```python
from build123d import *

# Parameters (mm, degrees)
SKETCH_4_W                   = 147
SKETCH_4_H                   = 102
EXTRUDE_1_DEPTH              = 26.5
PATTERN_LINEAR_3_COUNT       = 2
PATTERN_LINEAR_3_PITCH       = 44.45
PATTERN_LINEAR_3_COUNT_DIR2  = 2
PATTERN_LINEAR_3_PITCH_DIR2  = 95
SKETCH_10_W                  = 9
SKETCH_10_H                  = 5
CUT_EXTRUDE_1_DEPTH          = 103
SKETCH_12_W                  = 19.5
SKETCH_12_H                  = 5
CUT_EXTRUDE_2_DEPTH          = 103
CUT_EXTRUDE_3_DEPTH          = 4
CUT_EXTRUDE_4_DEPTH          = 1
CUT_EXTRUDE_7_DEPTH          = 5
SKETCH_16_W                  = 6
SKETCH_16_H                  = 3
CUT_EXTRUDE_8_DEPTH          = 4
PATTERN_LINEAR_4_COUNT       = 2
PATTERN_LINEAR_4_PITCH       = 41.61
PATTERN_LINEAR_4_COL_COUNT   = 2
PATTERN_LINEAR_4_COL_PITCH   = 101.6
MIRROR_2_COPY_1_SKETCH_W     = 6
MIRROR_2_COPY_1_SKETCH_H     = 3
MIRROR_2_COPY_1_DEPTH        = 4
MIRROR_2_COPY_2_SKETCH_W     = 6
MIRROR_2_COPY_2_SKETCH_H     = 3
MIRROR_2_COPY_2_DEPTH        = 4
PATTERN_LINEAR_1_COUNT       = 2
PATTERN_LINEAR_1_PITCH       = 41.61
PATTERN_LINEAR_1_COL_COUNT   = 2
PATTERN_LINEAR_1_COL_PITCH   = 101.6
SKETCH_17_R                  = 2.5
EXTRUDE_2_DEPTH              = 3
PATTERN_LINEAR_5_COUNT       = 2
PATTERN_LINEAR_5_PITCH       = 46.5
SKETCH_18_R                  = 2.5
EXTRUDE_3_DEPTH              = 3
DRAFT_1_ANGLE                = 2
SKETCH_19_W                  = 9
SKETCH_19_H                  = 81
CUT_EXTRUDE_9_DEPTH          = 1
SKETCH_21_W                  = 9
SKETCH_21_H                  = 42
CUT_EXTRUDE_10_DEPTH         = 4
SKETCH_22_W                  = 7
SKETCH_22_H                  = 41
SKETCH_22_H_2                = 40.5
CUT_EXTRUDE_11_DEPTH         = 6
HOLE_WIZARD_M3_3_D           = 2.5
HOLE_WIZARD_M3_3_DEPTH       = 8.5
HOLE_WIZARD_M3_3_CSINK_D     = 3.05
HOLE_WIZARD_M3_3_CSINK_ANGLE = 90
HOLE_WIZARD_M3_3_TIP         = 0.751075774
FILLET_1_R                   = 4


with BuildPart() as part:
    # 草图4 → 凸台-拉伸1 (new body)
    with BuildSketch(Plane(origin=(0, 0, 0), x_dir=(1, 0, 0), z_dir=(0, 1, 0))):
        Rectangle(SKETCH_4_W, SKETCH_4_H)
    extrude(amount=EXTRUDE_1_DEPTH)

    # 草图9 → M3 螺纹孔2 (revolve, cut)
    with BuildSketch(Plane(origin=(32.22, 0, 47.5), x_dir=(0, 0, -1), z_dir=(1, 0, 0))):
        Polygon((0, 0), (0, 8.251075774), (1.25, 7.5), (1.25, 0.275), (1.525, 0), align=None)
    hole_wizard_m3_2 = revolve(axis=Axis((32.22, -6.35, 47.5), (0, 1, 0)), mode=Mode.SUBTRACT)

    # 阵列(线性)3: Hole Wizard M3 _2 2 × 2
    with Locations(*[(-i * PATTERN_LINEAR_3_PITCH, 0, -j * PATTERN_LINEAR_3_PITCH_DIR2) for i in range(PATTERN_LINEAR_3_COUNT) for j in range(PATTERN_LINEAR_3_COUNT_DIR2) if (i, j) != (0, 0)]):
        add(hole_wizard_m3_2, mode=Mode.SUBTRACT)

    # 草图10 → 切除-拉伸1 (cut, through all)
    with BuildSketch(Plane.XY.offset(51)):
        with Locations((-69, 2.5)):
            Rectangle(SKETCH_10_W, SKETCH_10_H)
    extrude(amount=-CUT_EXTRUDE_1_DEPTH, mode=Mode.SUBTRACT)

    # 草图12 → 切除-拉伸2 (cut, through all)
    with BuildSketch(Plane.XY.offset(51)):
        with Locations((63.75, 2.5)):
            Rectangle(SKETCH_12_W, SKETCH_12_H)
    extrude(amount=-CUT_EXTRUDE_2_DEPTH, mode=Mode.SUBTRACT)

    # 草图13 → 切除-拉伸3 (cut)
    with BuildSketch(Plane.XZ.offset(-5)):
        Polygon((54, -51), (73.5, -31.5), (73.5, -51), align=None)
    extrude(amount=-CUT_EXTRUDE_3_DEPTH, mode=Mode.SUBTRACT)

    # 草图14 → 切除-拉伸4 (cut)
    with BuildSketch(Plane.XZ.offset(-5)):
        Polygon((54, 51), (73.5, 31.5), (73.5, 51), align=None)
    extrude(amount=-CUT_EXTRUDE_4_DEPTH, mode=Mode.SUBTRACT)

    # 草图15 → 切除-拉伸7 (cut)
    with BuildSketch(Plane.XZ):
        with BuildLine():
            Line((54, 47.7), (35.714281042, 47.7))
            ThreePointArc((35.714281042, 47.7), (32.22, 44), (28.725718958, 47.7))
            Line((28.725718958, 47.7), (-8.735718958, 47.7))
            ThreePointArc((-8.735718958, 47.7), (-12.23, 44), (-15.724281042, 47.7))
            Line((-15.724281042, 47.7), (-64.5, 47.7))
            Line((-64.5, 47.7), (-64.5, -47.7))
            Line((-64.5, -47.7), (-15.724281042, -47.7))
            ThreePointArc((-15.724281042, -47.7), (-12.23, -44), (-8.735718958, -47.7))
            Line((-8.735718958, -47.7), (28.725718958, -47.7))
            ThreePointArc((28.725718958, -47.7), (32.22, -44), (35.714281042, -47.7))
            Line((35.714281042, -47.7), (54, -47.7))
            Line((54, -47.7), (54, 47.7))
        make_face()
    extrude(amount=-CUT_EXTRUDE_7_DEPTH, mode=Mode.SUBTRACT)

    # 草图16 → 切除-拉伸8 (cut)
    with BuildSketch(Plane.XZ.offset(-5)):
        with Locations((45, 46.2)):
            Rectangle(SKETCH_16_W, SKETCH_16_H)
    cut_extrude_8 = extrude(amount=-CUT_EXTRUDE_8_DEPTH, mode=Mode.SUBTRACT)

    # 阵列(线性)4: 切除-拉伸8 ×2
    with Locations(*[(-i * PATTERN_LINEAR_4_PITCH, 0, 0) for i in range(1, PATTERN_LINEAR_4_COUNT)]):
        add(cut_extrude_8, mode=Mode.SUBTRACT)

    # 阵列(线性)4 col: 切除-拉伸8 ×2
    with Locations(*[(-i * PATTERN_LINEAR_4_COL_PITCH, 0, 0) for i in range(1, PATTERN_LINEAR_4_COL_COUNT)]):
        add(cut_extrude_8, mode=Mode.SUBTRACT)

    # 镜向2: 切除-拉伸8 across plane
    add(cut_extrude_8.mirror(Plane.XY), mode=Mode.SUBTRACT)

    # 镜向2 copy 1 sketch → 镜向2 copy 1 (cut)
    with BuildSketch(Plane(origin=(-41.61, 5, 0), x_dir=(1, 0, 0), z_dir=(0, -1, 0))):
        with Locations((45, -46.2)):
            Rectangle(MIRROR_2_COPY_1_SKETCH_W, MIRROR_2_COPY_1_SKETCH_H)
    extrude(amount=-MIRROR_2_COPY_1_DEPTH, mode=Mode.SUBTRACT)

    # 镜向2 copy 2 sketch → 镜向2 copy 2 (cut)
    with BuildSketch(Plane(origin=(-101.6, 5, 0), x_dir=(1, 0, 0), z_dir=(0, -1, 0))):
        with Locations((45, -46.2)):
            Rectangle(MIRROR_2_COPY_2_SKETCH_W, MIRROR_2_COPY_2_SKETCH_H)
    extrude(amount=-MIRROR_2_COPY_2_DEPTH, mode=Mode.SUBTRACT)

    # 草图7 → M3 螺纹孔1 (revolve, cut)
    with BuildSketch(Plane(origin=(45, 6.25, 51), x_dir=(0, -1, 0), z_dir=(1, 0, 0))):
        Polygon((0, 0), (0, 5.751075774), (1.25, 5), (1.25, 0.275), (1.525, 0), align=None)
    hole_wizard_m3_1 = revolve(axis=Axis((45, 6.25, 57.35), (0, 0, -1)), mode=Mode.SUBTRACT)

    # 阵列(线性)1: M3 螺纹孔1 ×2
    with Locations(*[(-i * PATTERN_LINEAR_1_PITCH, 0, 0) for i in range(1, PATTERN_LINEAR_1_COUNT)]):
        add(hole_wizard_m3_1, mode=Mode.SUBTRACT)

    # 阵列(线性)1 col: M3 螺纹孔1 ×2
    with Locations(*[(-i * PATTERN_LINEAR_1_COL_PITCH, 0, 0) for i in range(1, PATTERN_LINEAR_1_COL_COUNT)]):
        add(hole_wizard_m3_1, mode=Mode.SUBTRACT)

    # 镜向4: M3 螺纹孔1 across plane
    add(hole_wizard_m3_1.mirror(Plane.XY), mode=Mode.SUBTRACT)

    # 镜向4 copy 1 sketch → 镜向4 copy 1 (revolve, cut)
    with BuildSketch(Plane(origin=(3.39, 6.25, -51), x_dir=(0, -1, 0), z_dir=(1, 0, 0))):
        Polygon((0, 0), (0, -5.751075774), (1.25, -5), (1.25, -0.275), (1.525, 0), align=None)
    revolve(axis=Axis((3.39, 6.25, -57.35), (0, 0, -1)), mode=Mode.SUBTRACT)

    # 镜向4 copy 2 sketch → 镜向4 copy 2 (revolve, cut)
    with BuildSketch(Plane(origin=(-56.6, 6.25, -51), x_dir=(0, -1, 0), z_dir=(1, 0, 0))):
        Polygon((0, 0), (0, -5.751075774), (1.25, -5), (1.25, -0.275), (1.525, 0), align=None)
    revolve(axis=Axis((-56.6, 6.25, -57.35), (0, 0, -1)), mode=Mode.SUBTRACT)

    # 草图17 → 凸台-拉伸2 (add)
    with BuildSketch(Plane.XZ.offset(-5)):
        with Locations((57, 44)):
            Circle(SKETCH_17_R)
    extrude_2 = extrude(amount=EXTRUDE_2_DEPTH)

    # 阵列(线性)5: 凸台-拉伸2 ×2
    with Locations(*[(-i * PATTERN_LINEAR_5_PITCH, 0, 0) for i in range(1, PATTERN_LINEAR_5_COUNT)]):
        add(extrude_2)

    # 草图18 → 凸台-拉伸3 (add)
    with BuildSketch(Plane.XZ.offset(-5)):
        with Locations((10.5, -30)):
            Circle(SKETCH_18_R)
        with Locations((42.5, -16)):
            Circle(SKETCH_18_R)
        with Locations((59, -16)):
            Circle(SKETCH_18_R)
        with Locations((17, 9.5)):
            Circle(SKETCH_18_R)
    extrude(amount=EXTRUDE_3_DEPTH)

    # 拔模1
    draft_1_faces = [part.faces().sort_by_distance(p)[0] for p in [
        (8, 3.5, -30),
        (56.5, 3.5, -16),
        (40, 3.5, -16),
        (14.5, 3.5, 9.5),
        (8, 3.5, 44),
        (54.5, 3.5, 44),
    ]]
    draft(draft_1_faces, Plane(origin=(-73.5, 5, -51), x_dir=(0, 0, -1), z_dir=(0, -1, 0)), DRAFT_1_ANGLE)

    # 草图19 → 切除-拉伸9 (cut)
    with BuildSketch(Plane.XZ.offset(-5)):
        with Locations((69, 0)):
            Rectangle(SKETCH_19_W, SKETCH_19_H)
    extrude(amount=-CUT_EXTRUDE_9_DEPTH, mode=Mode.SUBTRACT)

    # 草图21 → 切除-拉伸10 (cut)
    with BuildSketch(Plane.XZ.offset(-5)):
        with Locations((69, -30)):
            Rectangle(SKETCH_21_W, SKETCH_21_H)
        with BuildLine():
            Line((73.5, 44), (69.5, 44))
            Line((69.5, 44), (69.5, 47.387489493))
            Line((69.5, 47.387489493), (66, 47.387489493))
            Line((66, 47.387489493), (66, 44))
            Line((66, 44), (64.5, 44))
            Line((64.5, 44), (64.5, -2.479274058))
            Line((64.5, -2.479274058), (68, -4.5))
            Line((68, -4.5), (68, -5.5))
            ThreePointArc((68, -5.5), (69.5, -7), (71, -5.5))
            Line((71, -5.5), (71, -4.5))
            Line((71, -4.5), (73.5, -2.5))
            Line((73.5, -2.5), (73.5, 44))
        make_face()
    extrude(amount=-CUT_EXTRUDE_10_DEPTH, mode=Mode.SUBTRACT)

    # 草图22 → 切除-拉伸11 (cut)
    with BuildSketch(Plane.XZ.offset(-9)):
        with Locations((68, 23.5)):
            Rectangle(SKETCH_22_W, SKETCH_22_H)
        with Locations((68, -29.25)):
            Rectangle(SKETCH_22_W, SKETCH_22_H_2)
    extrude(amount=-CUT_EXTRUDE_11_DEPTH, mode=Mode.SUBTRACT)

    # M3 螺纹孔3
    with Locations(Plane(origin=(0, 2, 0), x_dir=(-1, 0, 0), z_dir=(0, -1, 0))):
        with Locations((-57, -44), (-10.5, -44), (-17, -9.5), (-10.5, 30), (-42.5, 16), (-59, 16)):
            CounterSinkHole(HOLE_WIZARD_M3_3_D / 2, HOLE_WIZARD_M3_3_CSINK_D / 2, depth=HOLE_WIZARD_M3_3_DEPTH, counter_sink_angle=HOLE_WIZARD_M3_3_CSINK_ANGLE)
            with Locations((0, 0, -(HOLE_WIZARD_M3_3_DEPTH + HOLE_WIZARD_M3_3_TIP / 2))):  # 118° drill point
                Cone(0, HOLE_WIZARD_M3_3_D / 2, HOLE_WIZARD_M3_3_TIP, mode=Mode.SUBTRACT)

    # 圆角1
    fillet_1_edges = [part.edges().sort_by_distance(p)[0] for p in [
        (-73.5, 15.75, -51),
        (73.5, 17.75, -51),
        (73.5, 16.25, 51),
        (-73.5, 15.75, 51),
    ]]
    fillet(fillet_1_edges, radius=FILLET_1_R)


solid = part.part
```
For this review, take the finished solid that the model builds, in its own axes (mm). A direction names the side the tool comes from. Round coordinates to 2 decimals unless told otherwise and drop trailing zeros. Loops run counter-clockwise (first coordinate to the right, second up) from the corner with the lowest first, then second, coordinate; pieces in that order, holes last.
Q1. Insertion check: pin 1 Ø1.5 at (x, y) = (-56.6, 6.25) entering from -Z; pin 2 Ø7 at (x, y) = (45.5, 5) entering from +Z; pin 3 Ø0.9 at (y, z) = (7, -46) entering from +X; pin 4 Ø1.5 at (y, z) = (7, -46.5) entering from +X. Each pin has a flat end and moves straight along its axis. Give the tip position at first contact, or say it passes through.
Result sheet:
pin 1: stops at z = -44.7
pin 2: stops at z = 51
pin 3: stops at x = 59.45
pin 4: stops at x = 59.25
Q2. Machinability: for faces 1 (the face through (-59.6, 7, 46)), 2 (the face through (72.297, 16.394, 49.859)), which of the approach directions +Z, -Z, +X, -X, +Y, -Y give a long, thin tool a straight path to every point of the face, cutting with its end or side? Answer none if there is none.
Result sheet:
face 1: -Y
face 2: +Z, +X, +Y, -Y
Q3. Add section A-A on x = 22. Write out the cut boundary in (y, z), plus the area to 3 significant figures.
Result sheet:
outline: (0, -51) - (26.5, -51) - (26.5, 51) - (0, 51) - (0, 47.7) - (5, 47.7) - (5, -47.7) - (0, -47.7) - close
area: 2,230 mm2
Q4. Add section B-B on z = 16. Write out the cut boundary in (x, y).
Result sheet:
outline: (-73.5, 5) - (64.5, 5) - (64.5, 15) - (71.5, 15) - (71.5, 9) - (73.5, 9) - (73.5, 26.5) - (-73.5, 26.5) - close
Q5. Mouldability with a two-part tool opening along X and no side actions: class faces 3 (the face through (59.2, 5.5, 45.8)), 4 (the face through (-57, 9, -46)), 5 (the face through (59, 2, -18)) as +X half, -X half, draft (parallel to the pull), parting line (faces both ways), or undercut.
Result sheet:
face 3: +X half
face 4: undercut
face 5: draft
Q6. To check wall thickness, follow line 1 along Z through (x, y) = (10.5, 4); line 2 along X through (y, z) = (2, 47.5); line 3 along Z through (x, y) = (17, 4). State the ranges of each line that lie inside material, in increasing order.
Result sheet:
line 1: z = -51 to -47.7, -32.47 to -31.25, -28.75 to -27.53, 41.53 to 42.75, 45.25 to 46.47, 47.7 to 51
line 2: x = -15.73 to -13.48, -10.98 to -8.73, 28.72 to 30.97, 33.47 to 35.72
line 3: z = -51 to -47.7, 7.03 to 8.25, 10.75 to 11.97, 47.7 to 51
